CAD build for the part. Positions are in the model's coordinates, mm. Round coordinates to 2 decimals unless told otherwise and drop trailing zeros. Order: outer loops, then holes, each group sorted by start corner. A loop starts at its lowest first (then second) coordinate and runs counter-clockwise, first axis right, second up. Notation, with made-up numbers: M 16.5,26 L 69.5,26 A24 ccw 69.5,60 Z; hole C -5.5,-32 d5. An arc over 180 degrees is marked long. Answer as a JSON object with one key per item and string values.
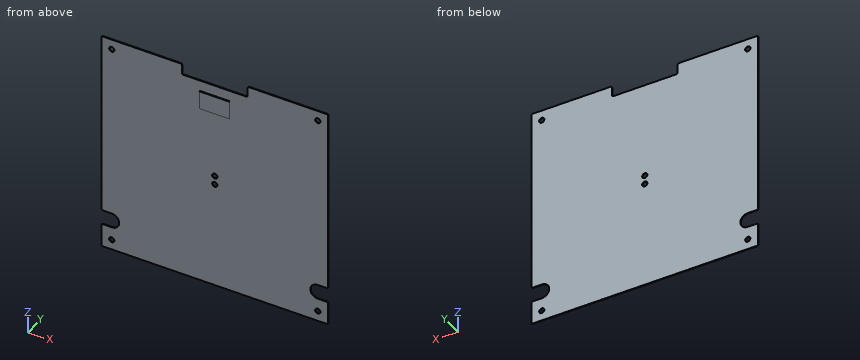
```python
from build123d import *

# Parameters (mm, degrees)
SKETCH1_W                = 304
SKETCH1_H                = 304
BOSS_EXTRUDE1_DEPTH      = 1
SKETCH2_W                = 88
SKETCH2_H                = 15
CUT_EXTRUDE1_DEPTH       = 215.962787477
FILLET1_R                = 2
F_7_0_7_DIAMETER_HOLE1_D = 7
SKETCH6_W                = 40
SKETCH6_H                = 25
BOSS_EXTRUDE2_DEPTH      = 1


with BuildPart() as part:
    # Sketch1 → Boss-Extrude1 (new body)
    with BuildSketch(Plane(origin=(0, 0, 0), x_dir=(1, 0, 0), z_dir=(0, 1, 0))):
        Rectangle(SKETCH1_W, SKETCH1_H)
    extrude(amount=BOSS_EXTRUDE1_DEPTH)

    # Sketch2 → Cut-Extrude1 (cut, through all)
    with BuildSketch(Plane(origin=(0, 1, 0), x_dir=(1, 0, 0), z_dir=(0, 1, 0))):
        with Locations((0, -144.5)):
            Rectangle(SKETCH2_W, SKETCH2_H)
        with BuildLine():
            Line((-152, 100), (-138, 100))
            ThreePointArc((-138, 100), (-128, 110), (-138, 120))
            Line((-138, 120), (-152, 120))
            Line((-152, 120), (-152, 100))
        make_face()
        with BuildLine():
            Line((152, 100), (138, 100))
            ThreePointArc((138, 100), (128, 110), (138, 120))
            Line((138, 120), (152, 120))
            Line((152, 120), (152, 100))
        make_face()
    extrude(amount=-CUT_EXTRUDE1_DEPTH, mode=Mode.SUBTRACT)

    # Fillet1
    fillet1_edges = [part.edges().sort_by_distance(p)[0] for p in [
        (44, 0.5, 152),
        (-44, 0.5, 152),
        (-44, 0.5, 137),
        (44, 0.5, 137),
        (-152, 0.5, -100),
        (-152, 0.5, -120),
        (152, 0.5, -120),
        (152, 0.5, -100),
        (-152, 0.5, -152),
        (152, 0.5, -152),
        (152, 0.5, 152),
        (-152, 0.5, 152),
    ]]
    fillet(fillet1_edges, radius=FILLET1_R)

    # Ø7.0 (7) Diameter Hole1 (through all)
    with Locations(Plane(origin=(0, 1, 0), x_dir=(1, 0, 0), z_dir=(0, 1, 0))):
        with Locations((-138, -138), (138, 138), (-138, 138), (138, -138), (0, -6), (0, 6)):
            Hole(F_7_0_7_DIAMETER_HOLE1_D / 2)

    # Sketch6 → Boss-Extrude2 (add)
    with BuildSketch(Plane.XZ):
        with Locations((0, 109.5)):
            Rectangle(SKETCH6_W, SKETCH6_H)
    extrude(amount=BOSS_EXTRUDE2_DEPTH)


solid = part.part
```
Item 1: Wall check: line 1 along Z through (x, y) = (138, 0.75); line 2 along X through (y, z) = (0.3, -138); line 3 along Z through (x, y) = (0, 0.7). Give the ranges that are in metal, low to high. Write a range as [from, to].
Worked answers:
{"line 1": "z = [-152, -141.5], [-134.5, -120], [-100, 134.5], [141.5, 152]", "line 2": "x = [-152, -141.5], [-134.5, 134.5], [141.5, 152]", "line 3": "z = [-152, -9.5], [-2.5, 2.5], [9.5, 137]"}
Item 2: Saw through at B-B on z = -138. List the corners of the cut face in (x, y), and give its area (3 significant figures).
Worked answers:
{"outline": "M -152,0 L -141.5,0 L -141.5,1 L -152,1 Z; M -134.5,0 L 134.5,0 L 134.5,1 L -134.5,1 Z; M 141.5,0 L 152,0 L 152,1 L 141.5,1 Z", "area": "290 mm2"}
Item 3: Saw through at A-A on x = 0. List the corners of the cut face in (y, z).
Worked answers:
{"outline": "M -1,97 L 0,97 L 0,9.5 L 1,9.5 L 1,137 L 0,137 L 0,122 L -1,122 Z; M 0,-152 L 1,-152 L 1,-9.5 L 0,-9.5 Z; M 0,-2.5 L 1,-2.5 L 1,2.5 L 0,2.5 Z"}
Item 4: Drop flat-ended pins along their axis: pin 1 Ø0.8 at (y, z) = (-0.5, 110.5) entering from -X; pin 2 Ø11 at (x, z) = (-138, 138) entering from -Y; pin 3 Ø4 at (x, z) = (0, -6) entering from +Y (3 decimals); pin 4 Ø1.1 at (x, y) = (-9, -0.5) entering from +Z. Give the stop position or say it passes through.
Worked answers:
{"pin 1": "stops at x = -20", "pin 2": "stops at y = 0", "pin 3": "passes through", "pin 4": "stops at z = 137"}
Item 5: Saw through at C-C on z = 6. List the corners of the cut face in (x, y), and give its area (3 significant figures).
Worked answers:
{"outline": "M -152,0 L -3.5,0 L -3.5,1 L -152,1 Z; M 3.5,0 L 152,0 L 152,1 L 3.5,1 Z", "area": "297 mm2"}
Item 6: Saw through at D-D on x = 31.5. List the corners of the cut face in (y, z), and give its area (3 significant figures).
Worked answers:
{"outline": "M 0,-152 L 1,-152 L 1,137 L 0,137 Z", "area": "289 mm2"}
